Source: three-view drawing plus pictorial views. Frame: mm from the lowest corner of the part. A direction names the side the tool comes from. Coordinates: 2 decimals unless noted, no trailing zeros. Write each loop counter-clockwise with the first axis right and the second up, starting at its lowest first coordinate (ties: lowest second). Pieces come first, ordered by that corner, then holes. Notation, with made-up numbers: (-39, 70.25) - (-30, 70.25) arc R26 ccw to (-30, 104.25) - close; hole circle Ø1 at (15.5, 22). An arc over 180 degrees is marked (long way). Put each result on its own line as item: value.
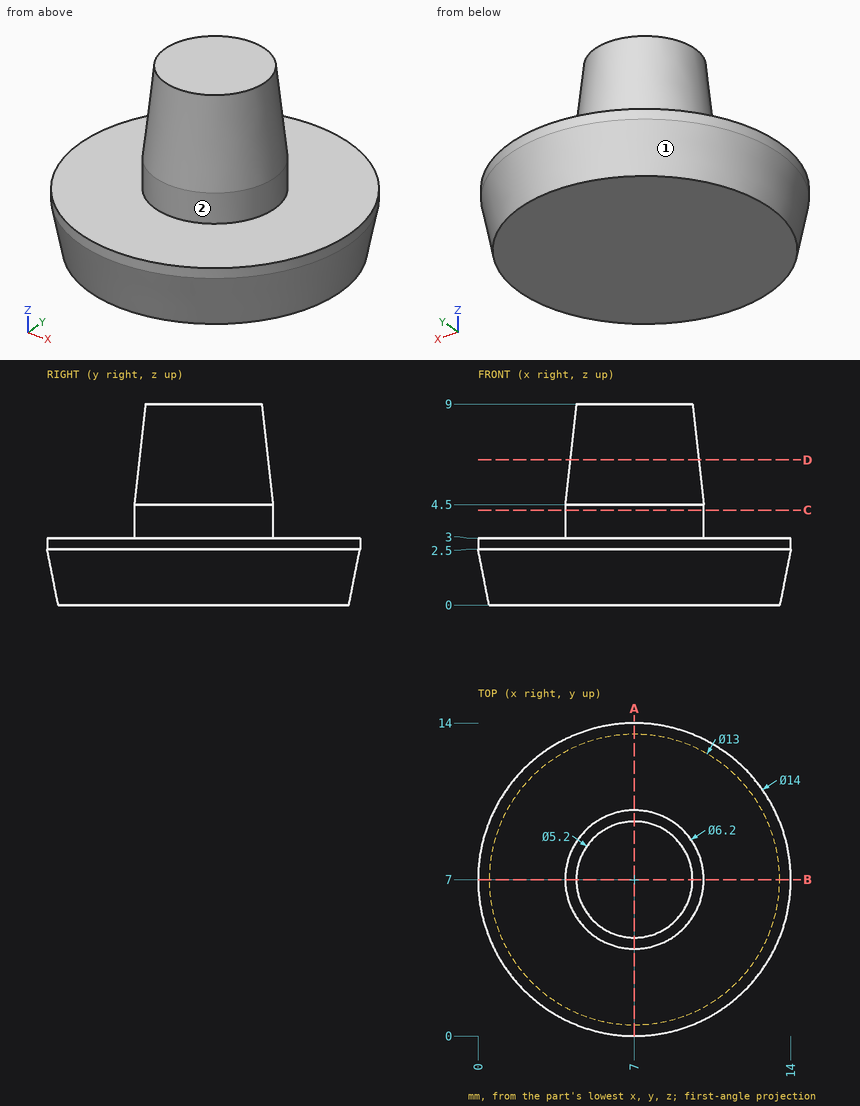
1. Set-up query: the marked faces 1 and 2. Return all of +Z, -Z, +X, -X, +Y, -Y with unobstructed straight access to the full face (end or side cutting, diameter ignored); none if empty.
Answer below:
face 1: -Z
face 2: +Z
2. Section query A-A (x = 7). Return loops of the section in (y, z).
Answer below:
outline: (0, 2.5) - (0.5, 0) - (13.5, 0) - (14, 2.5) - (14, 3) - (10.1, 3) - (10.1, 4.5) - (9.6, 9) - (4.4, 9) - (3.9, 4.5) - (3.9, 3) - (0, 3) - close
3. Ray query, probe 1 along Z at (x, y) = (9.75, 9.25); probe 2 along Y at (x, z) = (7, 3.25); probe 3 along X at (y, z) = (7.25, 6.75). Return the intervals inside material, ascending. Write a range as from..to.
Answer below:
probe 1: z = 0..3
probe 2: y = 3.9..10.1
probe 3: x = 4.16..9.84
4. Pin query (flat end, axial travel): pin 1 Ø1 at (y, z) = (3.5, 6.5) entering from -X; pin 2 Ø3 at (y, z) = (10.5, 8) entering from +X; pin 3 Ø5 at (y, z) = (9.5, 8) entering from -X; pin 4 Ø3 at (y, z) = (12.5, 1) entering from -X. Return the tip coordinate at first contact, or that it passes through.
Answer below:
pin 1: passes through
pin 2: stops at x = 8.85
pin 3: stops at x = 4.17
pin 4: stops at x = 1.56
5. Section query D-D (z = 6.5). Return loops of the section in (x, y).
Answer below:
outline: circle Ø5.76 at (7, 7)
6. Section query C-C (z = 4.25). Return loops of the section in (x, y), then the cut area to 3 significant figures.
Answer below:
outline: circle Ø6.2 at (7, 7)
area: 30.2 mm²
